Source: CAD feature listing. Evaluate the final solid. Frame: model axes, mm. Face numbers are marked on the shaded views. A direction names the side the tool comes from. Give positions to 0.01 mm unless a question says otherwise; leave off trailing zeros. Order: outer loops, then holes, each group sorted by start corner. A loop starts at its lowest first (then second) coordinate and runs counter-clockwise, first axis right, second up. Notation, with made-up numbers: M -39.75,4.5 L -7.75,4.5 A20 cw -7.75,25.5 Z; hole C 72,8 d5. An arc over 180 degrees is marked long. Return JSON: item names as keys, results as strings.
from build123d import *

# Parameters (mm, degrees)
SKETCH3_R           = 3.96875
SKETCH3_R_2         = 3.175
BOSS_EXTRUDE4_DEPTH = 10.16
SKETCH5_W           = 15.875
SKETCH5_H           = 13.97
CUT_EXTRUDE3_DEPTH  = 5.08
FILLET1_R           = 3.81
SKETCH6_R           = 5.05
CUT_EXTRUDE4_DEPTH  = 3.3


with BuildPart() as part:
    # Sketch3 → Boss-Extrude4 (new body)
    with BuildSketch(Plane(origin=(0, 0, 0), x_dir=(1, 0, 0), z_dir=(0, 1, 0))):
        with BuildLine():
            Line((54.2925, 31.75), (-12.3825, 31.75))
            Line((-12.3825, 31.75), (-7.863361559, -1.082336008))
            ThreePointArc((-7.863361559, -1.082336008), (-3.056289676, -7.325503373), (4.7625, -6.35))
            Line((4.7625, -6.35), (41.91, -6.35))
            ThreePointArc((41.91, -6.35), (45.967580476, -4.884520517), (48.152310263, -1.164501002))
            Line((48.152310263, -1.164501002), (54.2925, 31.75))
        make_face()
        Circle(SKETCH3_R, mode=Mode.SUBTRACT)
        with Locations((-4.445, 22.86)):
            Circle(SKETCH3_R, mode=Mode.SUBTRACT)
        with Locations((46.355, 22.86)):
            Circle(SKETCH3_R, mode=Mode.SUBTRACT)
        with Locations((41.91, 0)):
            Circle(SKETCH3_R_2, mode=Mode.SUBTRACT)
        with BuildLine():
            Line((38.735, 8.89), (38.735, 27.305))
            ThreePointArc((38.735, 27.305), (38.363025612, 28.203025612), (37.465, 28.575))
            Line((37.465, 28.575), (4.445, 28.575))
            ThreePointArc((4.445, 28.575), (3.546974388, 28.203025612), (3.175, 27.305))
            Line((3.175, 27.305), (3.175, 8.89))
            ThreePointArc((3.175, 8.89), (3.546974388, 7.991974388), (4.445, 7.62))
            Line((4.445, 7.62), (37.465, 7.62))
            ThreePointArc((37.465, 7.62), (38.363025612, 7.991974388), (38.735, 8.89))
        make_face(mode=Mode.SUBTRACT)
        with BuildLine():
            Line((20.32, 3.175), (14.605, 3.175))
            ThreePointArc((14.605, 3.175), (11.43, 0), (14.605, -3.175))
            Line((14.605, -3.175), (20.32, -3.175))
            ThreePointArc((20.32, -3.175), (22.498043553, -2.310140965), (23.489504023, -0.186733089))
            Line((23.489504023, -0.186733089), (21.228562514, 3.04222602))
            ThreePointArc((21.228562514, 3.04222602), (20.779106407, 3.141631154), (20.32, 3.175))
        make_face(mode=Mode.SUBTRACT)
        with BuildLine():
            Line((46.58698696, 4.295147609), (48.697586564, 15.60902157))
            ThreePointArc((48.697586564, 15.60902157), (45.177345011, 15.331552037), (41.91, 16.670785591))
            Line((41.91, 16.670785591), (41.91, 6.35))
            ThreePointArc((41.91, 6.35), (44.464242812, 5.81363429), (46.58698696, 4.295147609))
        make_face(mode=Mode.SUBTRACT)
        with BuildLine():
            Line((-6.080523252, 4.592563226), (-7.642900683, 15.943510195))
            ThreePointArc((-7.642900683, 15.943510195), (-3.723164456, 15.274266453), (0, 16.670785591))
            Line((0, 16.670785591), (0, 7.62))
            ThreePointArc((0, 7.62), (-3.396252951, 6.82128037), (-6.080523252, 4.592563226))
        make_face(mode=Mode.SUBTRACT)
        with BuildLine():
            Line((36.410738686, -3.175), (27.305, -3.175))
            Line((27.305, -3.175), (27.305, 3.81))
            Line((27.305, 3.81), (36.83, 3.81))
            ThreePointArc((36.83, 3.81), (35.571407985, 0.380461907), (36.410738686, -3.175))
        make_face(mode=Mode.SUBTRACT)
    extrude(amount=BOSS_EXTRUDE4_DEPTH)

    # Sketch5 → Cut-Extrude3 (cut)
    with BuildSketch(Plane(origin=(0, 10.16, 0), x_dir=(1, 0, 0), z_dir=(0, 1, 0))):
        with Locations((17.4625, 0.635)):
            Rectangle(SKETCH5_W, SKETCH5_H)
    extrude(amount=-CUT_EXTRUDE3_DEPTH, mode=Mode.SUBTRACT)

    # Fillet1
    fillet1_edges = [part.edges().sort_by_distance(p)[0] for p in [
        (-12.3825, 5.08, -31.75),
        (54.2925, 5.08, -31.75),
    ]]
    fillet(fillet1_edges, radius=FILLET1_R)

    # Sketch6 → Cut-Extrude4 (cut)
    with BuildSketch(Plane(origin=(0, 10.16, 0), x_dir=(1, 0, 0), z_dir=(0, 1, 0))):
        Circle(SKETCH6_R)
    extrude(amount=-CUT_EXTRUDE4_DEPTH, mode=Mode.SUBTRACT)


solid = part.part
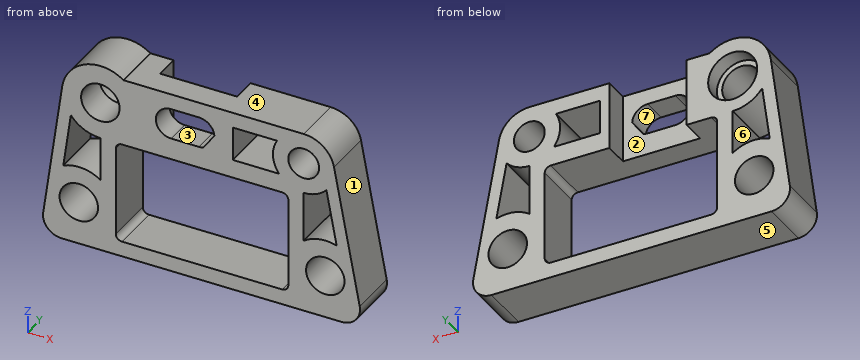
1. Set-up query: the marked faces 1, 2 and 3. Return all of +Z, -Z, +X, -X, +Y, -Y with unobstructed straight access to the full face (end or side cutting, diameter ignored); none if empty.
Evaluation:
{"face 1": "+Z, +X, +Y, -Y", "face 2": "+Z, +Y", "face 3": "+Y, -Y"}
2. Draft query along Z for the marked faces 4, 5, 6 and 7. Return one class per face: pulls with the +Z half, pulls with the -Z half, needs draft (parallel to the pull), parting line crosses it, or undercut.
Evaluation:
{"face 4": "pulls with the +Z half", "face 5": "pulls with the -Z half", "face 6": "undercut", "face 7": "undercut"}
3. Section query B-B (z = -22.86). Return loops of the section in (x, y) (3 decimals).
Evaluation:
{"outline": "M -11.159,0 L -8.414,0 L -8.414,10.16 L -11.159,10.16 Z; M -0.476,0 L 3.175,0 L 3.175,10.16 L -0.476,10.16 Z; M 38.735,0 L 42.386,0 L 42.386,10.16 L 38.735,10.16 Z; M 50.324,0 L 52.634,0 L 52.634,10.16 L 50.324,10.16 Z"}
4. Ray query, probe 1 along Z at (x, y) = (33.5, 6) (3 decimals); probe 2 along X at (y, z) = (7.75, 0) (3 decimals); probe 3 along Z at (x, y) = (26.5, 3.25) (3 decimals). Return the intervals inside material, ascending.
Evaluation:
{"probe 1": "z = -31.75 to -28.575, -7.62 to -3.81, 3.175 to 6.35", "probe 2": "x = -8.012 to -5.05, 5.05 to 9.525, 25.4 to 27.305, 35.56 to 38.735, 45.085 to 48.37", "probe 3": "z = -31.75 to -28.575, -7.62 to 6.35"}
5. Section query D-D (y = 5.75). State how many separate pieces and enclosed holes the cut face has, then the cut area to 3 significant figures.
Evaluation:
{"separate pieces": "1", "enclosed holes": "7", "area": "971 mm^2"}
6. First-contact query: pin 1 (1 mm diameter, centred on y = 2, z = -5.5, fed in from -X); pin 2 (1.5 mm diameter, centred on x = 17.5, y = 2, fed in from +Z); pin 3 (4 mm diameter, centred on y = 2, z = 2.5, fed in from -X); pin 4 (12.5 mm diameter, centred on x = 46.355, z = -22.86, fed in from +Y). Flat tips, straight axial feed; report the tip coordinate or a pass-through.
Evaluation:
{"pin 1": "stops at x = -8.84", "pin 2": "stops at z = 6.35", "pin 3": "stops at x = -7.94", "pin 4": "stops at y = 10.16"}
7. Section query A-A (x = 18.5). Return loops of the section in (y, z) (3 decimals), then the cut area to 3 significant figures.
Evaluation:
{"outline": "M 0,-31.75 L 10.16,-31.75 L 10.16,-28.575 L 0,-28.575 Z; M 0,-7.62 L 5.08,-7.62 L 5.08,-3.175 L 0,-3.175 Z; M 0,3.175 L 5.08,3.175 L 5.08,6.35 L 0,6.35 Z", "area": "71.0 mm^2"}
8. Section query C-C (x = 41). Return loops of the section in (y, z).
Evaluation:
{"outline": "M 0,-31.75 L 10.16,-31.75 L 10.16,-3.04 L 0,-3.04 Z; M 0,3.04 L 10.16,3.04 L 10.16,6.35 L 0,6.35 Z"}
